from build123d import *

# Parameters (mm, degrees)
EXTRUDE_1_DEPTH = 3
EXTRUDE_2_DEPTH = 3.5
FILLET_3_R      = 1


with BuildPart() as part:
    # ｽｹｯﾁ1 → ﾎﾞｽ - 押し出し1 (new body)
    with BuildSketch(Plane(origin=(0, 0, 0), x_dir=(1, 0, 0), z_dir=(0, 1, 0))):
        Polygon((0, 0), (7, 0), (12, 0), (19, 0), (19, 73.05), (0, 73.05), align=None)
    extrude(amount=EXTRUDE_1_DEPTH)

    # ｽｹｯﾁ2 → ﾎﾞｽ - 押し出し2 (add)
    with BuildSketch(Plane(origin=(0, 3, 0), x_dir=(1, 0, 0), z_dir=(0, 1, 0))):
        Polygon((1.4, 0), (3, 5.5), (3, 7.5), (0, 7.5), (0, 0), align=None)
        Polygon((0, 15.5), (3.275, 15.5), (3.275, 70.05), (15.725, 70.05), (15.725, 0), (19, 0), (19, 73.05), (0, 73.05), align=None)
    extrude(amount=EXTRUDE_2_DEPTH)

    # ﾌｨﾚｯﾄ3
    fillet_3_edges = [part.edges().sort_by_distance(p)[0] for p in [
        (0, 3.25, -73.05),
        (19, 3.25, -73.05),
        (19, 3.25, 0),
        (0, 3.25, 0),
    ]]
    fillet(fillet_3_edges, radius=FILLET_3_R)


solid = part.part
Can you work these out from the model? Positions are in its coordinate system, mm. A direction names the side the tool comes from. Coordinates: 2 decimals unless noted, no trailing zeros. Write each loop counter-clockwise with the first axis right and the second up, starting at its lowest first coordinate (ties: lowest second). Pieces come first, ordered by that corner, then holes. Notation, with made-up numbers: (-12, -18.5) - (-4, -18.5) arc R31 ccw to (-4, 12.5) - close; hole circle Ø3 at (-15, 81). An arc over 180 degrees is marked (long way). Return JSON: item names as keys, results as strings. Group by question number.
Item 1: We'd pull the mould along Z, two halves only. Please class faces 1 (the face through (15.725, 5, -36)), 2 (the face through (2, 5, -15.5)), 3 (the face through (9, 5, -70.05)): pulls with the +Z half, pulls with the -Z half, needs draft (parallel to the pull), parting line crosses it, or undercut.
Item 2: If we section it at C-C (x = 12): Write out the boundary of the cut face in (y, z), then the cut area to 3 significant figures.
Item 3: I'm going to push a flat-ended pin straight in: pin 1 Ø6 at (x, z) = (9.5, -36.5) entering from +Y. Where does the tip first touch, or does it pass through?
Item 4: Please list where these lines run through material, in increasing order: probe 1 along X at (y, z) = (5, -25) (3 decimals); probe 2 along Z at (x, y) = (8.25, 4); probe 3 along Y at (x, z) = (5.75, -44).
Item 5: If we section it at A-A (y = 5.5): Write out the boundary of the cut face in (x, z) (3 decimals).
Item 6: If we section it at B-B (z = -52.5): Write out the boundary of the cut face in (x, y) (3 decimals), then the cut area to 3 significant figures.
Item 7: Which directions (+Z, -Z, +X, -X, +Y, -Y) give clear straight access to the entire face, cutting with the end or side of a thin tool? Please do faces 4 (the face through (9, 2, 0)), 5 (the face through (3.275, 5, -42)), 6 (the face through (2, 5, -7.5)).
Return value:
{
 "1": {"face 1": "needs draft", "face 2": "undercut", "face 3": "pulls with the +Z half"},
 "2": {"outline": "(0, -73.05) - (6.5, -73.05) - (6.5, -70.05) - (3, -70.05) - (3, 0) - (0, 0) - close", "area": "230 mm^2"},
 "3": {"pin 1": "stops at y = 3"},
 "4": {"probe 1": "x = 0 to 3.275, 15.725 to 19", "probe 2": "z = -73.05 to -70.05", "probe 3": "y = 0 to 3"},
 "5": {"outline": "(0, -72.05) arc R1 ccw to (1, -73.05) - (18, -73.05) arc R1 ccw to (19, -72.05) - (19, -1) arc R1 ccw to (18, 0) - (15.725, 0) - (15.725, -70.05) - (3.275, -70.05) - (3.275, -15.5) - (0, -15.5) - close; (0, -7.5) - (3, -7.5) - (3, -5.5) - (1.4, 0) - (1, 0) arc R1 ccw to (0, -1) - close"},
 "6": {"outline": "(0, 0) - (19, 0) - (19, 6.5) - (15.725, 6.5) - (15.725, 3) - (3.275, 3) - (3.275, 6.5) - (0, 6.5) - close", "area": "79.9 mm^2"},
 "7": {"face 4": "+Z, +X, -X, +Y, -Y", "face 5": "+Z, +Y", "face 6": "-X, +Y"}
}
